Work out the finished part from the listing and answer in its coordinate system (mm). A direction names the side the tool comes from. Coordinates: 2 decimals unless noted, no trailing zeros. Order: outer loops, then holes, each group sorted by start corner. A loop starts at its lowest first (then second) coordinate and runs counter-clockwise, first axis right, second up. Notation, with made-up numbers: (62, 62.5) -> (100, 62.5) arc R7 cw to (100, 66.5) -> close; hole circle Ø11 at (8.25, -25.5). An arc over 180 degrees is marked (long way). Use one line per item in the form item = value.
from build123d import *

# Parameters (mm, degrees)
SKETCH1_W               = 68
SKETCH1_H               = 44
BOSS_EXTRUDE1_DEPTH     = 2
SKETCH2_R               = 2
CUT_EXTRUDE1_DEPTH      = 2
SKETCH3_W               = 12
SKETCH3_H               = 23
CUT_EXTRUDE2_DEPTH      = 2
SKETCH4_W               = 3
SKETCH4_H               = 23
BOSS_EXTRUDE2_DEPTH     = 2
SKETCH5_W               = 3
SKETCH5_H               = 21.5
BOSS_EXTRUDE3_DEPTH     = 6.5
SKETCH6_W               = 4
SKETCH6_H               = 2
BOSS_EXTRUDE4_DEPTH     = 10
CUT_EXTRUDE3_DEPTH      = 20
CUT_EXTRUDE3_DEPTH_BACK = 20
SKETCH7_W               = 8.75
SKETCH7_H               = 6.5
SKETCH7_W_2             = 10.25
CHAMFER1_SIZE           = 2
SKETCH8_W               = 6
SKETCH8_H               = 12
CUT_EXTRUDE4_DEPTH      = 20
CHAMFER2_SIZE           = 1
CHAMFER3_SIZE           = 1
CHAMFER4_SIZE           = 2


with BuildPart() as part:
    # Sketch1 → Boss-Extrude1 (new body)
    with BuildSketch(Plane(origin=(0, 0, 0), x_dir=(1, 0, 0), z_dir=(0, 1, 0))):
        with Locations((4.391941392, -7.446886447)):
            Rectangle(SKETCH1_W, SKETCH1_H)
    extrude(amount=BOSS_EXTRUDE1_DEPTH)

    # Sketch2 → Cut-Extrude1 (cut)
    with BuildSketch(Plane(origin=(0, 2, 0), x_dir=(1, 0, 0), z_dir=(0, 1, 0))):
        with Locations(Location((-22.108058608, 7.253113553, 0), (0, 0, 270))):
            Circle(SKETCH2_R)
        with Locations(Location((31.091941392, 7.253113553, 0), (0, 0, 270))):
            Circle(SKETCH2_R)
        with Locations(Location((31.091941392, -22.146886447, 0), (0, 0, 270))):
            Circle(SKETCH2_R)
        with Locations(Location((-22.108058608, -22.146886447, 0), (0, 0, 270))):
            Circle(SKETCH2_R)
    extrude(amount=-CUT_EXTRUDE1_DEPTH, mode=Mode.SUBTRACT)

    # Sketch3 → Cut-Extrude2 (cut)
    with BuildSketch(Plane(origin=(0, 2, 0), x_dir=(1, 0, 0), z_dir=(0, 1, 0))):
        with Locations((32.391941392, -7.446886447)):
            Rectangle(SKETCH3_W, SKETCH3_H)
    extrude(amount=-CUT_EXTRUDE2_DEPTH, mode=Mode.SUBTRACT)

    # Sketch4 → Boss-Extrude2 (add)
    with BuildSketch(Plane(origin=(0, 2, 0), x_dir=(1, 0, 0), z_dir=(0, 1, 0))):
        with Locations((36.891941392, -7.446886447)):
            Rectangle(SKETCH4_W, SKETCH4_H)
    extrude(amount=-BOSS_EXTRUDE2_DEPTH)

    # Sketch5 → Boss-Extrude3 (add)
    with BuildSketch(Plane(origin=(0, 2, 0), x_dir=(1, 0, 0), z_dir=(0, 1, 0))):
        with Locations((36.891941392, -6.696886447)):
            Rectangle(SKETCH5_W, SKETCH5_H)
        with Locations((24.891941392, -8.196886447)):
            Rectangle(SKETCH5_W, SKETCH5_H)
    extrude(amount=BOSS_EXTRUDE3_DEPTH)

    # Sketch6 → Boss-Extrude4 (add)
    with BuildSketch(Plane(origin=(26.391941392, 0, 0), x_dir=(0, 0, -1), z_dir=(1, 0, 0))):
        with Locations((-8.196886447, 7.5)):
            Rectangle(SKETCH6_W, SKETCH6_H)
    extrude(amount=BOSS_EXTRUDE4_DEPTH)

    # Sketch7 → Cut-Extrude3 (cut, two sides: drawn at the far end of the back side and taken through both)
    with BuildSketch(Plane(origin=(26.391941392, 0, 0), x_dir=(0, 0, -1), z_dir=(1, 0, 0)).offset(-CUT_EXTRUDE3_DEPTH_BACK)):
        with Locations((-14.571886447, 5.25)):
            Rectangle(SKETCH7_W, SKETCH7_H)
        with Locations((-1.071886447, 5.25)):
            Rectangle(SKETCH7_W_2, SKETCH7_H)
    extrude(amount=CUT_EXTRUDE3_DEPTH + CUT_EXTRUDE3_DEPTH_BACK, mode=Mode.SUBTRACT)

    # Chamfer1
    chamfer1_edges = [part.edges().sort_by_distance(p)[0] for p in [
        (24.891941392, 2, 10.196886447),
        (36.891941392, 2, 10.196886447),
        (24.891941392, 2, 6.196886447),
        (36.891941392, 2, 6.196886447),
    ]]
    chamfer(chamfer1_edges, length=CHAMFER1_SIZE)

    # Sketch8 → Cut-Extrude4 (cut)
    with BuildSketch(Plane(origin=(0, 2, 0), x_dir=(1, 0, 0), z_dir=(0, 1, 0))):
        with Locations((-26.608058608, -7.446886447)):
            Rectangle(SKETCH8_W, SKETCH8_H)
    extrude(amount=-CUT_EXTRUDE4_DEPTH, mode=Mode.SUBTRACT)

    # Chamfer2
    chamfer2_edges = [part.edges().sort_by_distance(p)[0] for p in [
        (-29.608058608, 1, 13.446886447),
        (-29.608058608, 1, 1.446886447),
    ]]
    chamfer(chamfer2_edges, length=CHAMFER2_SIZE)

    # Chamfer3
    chamfer3_edges = [part.edges().sort_by_distance(p)[0] for p in [
        (30.891941392, 6.5, 10.196886447),
    ]]
    chamfer(chamfer3_edges, length=CHAMFER3_SIZE)

    # Chamfer4
    chamfer4_edges = [part.edges().sort_by_distance(p)[0] for p in [
        (-29.608058608, 1, -14.553113553),
        (38.391941392, 1, -14.553113553),
        (38.391941392, 1, 29.446886447),
        (-29.608058608, 1, 29.446886447),
    ]]
    chamfer(chamfer4_edges, length=CHAMFER4_SIZE)


solid = part.part
(1) Section B-B on z = 11.5 is taken. Write down the section's boundary in (x, y).
Data:
outline = (-23.61, 0) -> (26.39, 0) -> (26.39, 2.7) -> (23.39, 2.7) -> (23.39, 2) -> (-23.61, 2) -> close; (35.39, 0) -> (38.39, 0) -> (38.39, 2.7) -> (35.39, 2.7) -> close
(2) Each of these flat-tipped pins is pushed along its axis until it touches: P1, Ø2, axis at x = 15, z = 18.5, coming from the +Y side; P2, Ø2.5, axis at x = -22.11, z = -7.25, coming from the +Y side; P3, Ø3.5, axis at x = 29.5, y = 6, coming from the +Z side; P4, Ø1.4, axis at x = 31.5, y = 6.5, coming from the -Z side. Where does it stop, or does it pass through?
Data:
P1 = 2
P2 = through
P3 = 10.2
P4 = 6.2
(3) The mould has two halves that part along Z. Classify faces 5 (the flat face through (31, 6.5, 8)), 6 (the flat face through (37.38, 0.99, 28.46)), 7 (the flat face through (-26, 1, 1.447)): released by +Z, released by -Z, zero draft, split by the parting line, or undercut.
Data:
face_5 = zero draft
face_6 = released by +Z
face_7 = undercut
(4) Which of the six approach directions +Z, -Z, +X, -X, +Y, -Y give full straight-line access (tool end or side, diameter ignored) to faces 1 (the flat face through (23.392, 5, 8)), 2 (the flat face through (-23.608, 1, 8)), 3 (the flat face through (35.392, 2, 8)), 4 (the flat face through (31, 1, 18.947))?
Data:
face_1 = +Z, -Z, -X, +Y
face_2 = -X, +Y, -Y
face_3 = -Y
face_4 = +Y, -Y
(5) Section A-A on y = 4.75 is taken. Write down the section's boundary in (x, z).
Data:
outline = (23.39, 6.2) -> (26.39, 6.2) -> (26.39, 10.2) -> (23.39, 10.2) -> close; (35.39, 6.2) -> (38.39, 6.2) -> (38.39, 10.2) -> (35.39, 10.2) -> close
(6) Section C-C on x = 24.5 is taken. Write down the section's boundary in (y, z).
Data:
outline = (0, -14.55) -> (2, -14.55) -> (2, 4.2) -> (4, 6.2) -> (8.5, 6.2) -> (8.5, 10.2) -> (4, 10.2) -> (2, 12.2) -> (2, 29.45) -> (0, 29.45) -> close
(7) Section D-D on y = 1.25 is taken. Write down the section's boundary in (x, z).
Data:
outline = (-29.61, -12.55) -> (-27.61, -14.55) -> (36.39, -14.55) -> (38.39, -12.55) -> (38.39, 27.45) -> (36.39, 29.45) -> (-27.61, 29.45) -> (-29.61, 27.45) -> (-29.61, 14.45) -> (-28.61, 13.45) -> (-23.61, 13.45) -> (-23.61, 1.45) -> (-28.61, 1.45) -> (-29.61, 0.45) -> close; hole circle Ø4 at (-22.11, -7.25); hole circle Ø4 at (-22.11, 22.15); hole (26.39, -4.05) -> (35.39, -4.05) -> (35.39, 18.95) -> (26.39, 18.95) -> close; hole circle Ø4 at (31.09, -7.25); hole circle Ø4 at (31.09, 22.15)
(8) Straight lines are drawn through the part: line 1 along X through (y, z) = (0.75, -5.5); line 2 along X through (y, z) = (1, 11); line 3 along Z through (x, y) = (27, 1.75). For each, find the intervals that lie inside material, in ascending order.
Data:
line_1 = -29.61 to -23.07, -21.15 to 30.13, 32.05 to 38.39
line_2 = -23.61 to 26.39, 35.39 to 38.39
line_3 = -14.55 to -4.05, 18.95 to 29.45
